Model file for the job. Use its own axes, mm. A direction names the side the tool comes from. Coordinates: 2 decimals unless noted, no trailing zeros. Write each loop counter-clockwise with the first axis right and the second up, starting at its lowest first coordinate (ties: lowest second). Pieces come first, ordered by that corner, then holes. Notation, with made-up numbers: M -22.75,50 L -0.75,50 A17 cw -0.75,63 Z; hole C -19.5,77.25 d5. An arc over 180 degrees is marked long. Answer in a Markdown table with one row per item. Add a question column.
```python
from build123d import *

# Parameters (mm, degrees)
SALIENTE_EXTRUIR1_DEPTH = 11.5
CORTAR_EXTRUIR1_START   = -5
CROQUIS2_R              = 2.1
CORTAR_EXTRUIR1_DEPTH   = 5
CROQUIS3_R              = 4.5
CORTAR_EXTRUIR2_DEPTH   = 0.5
CROQUIS4_R              = 3
CORTAR_EXTRUIR3_DEPTH   = 0.2
CROQUIS5_R              = 2.1
CROQUIS5_R_2            = 1.6
SALIENTE_EXTRUIR2_DEPTH = 0.6
CORTAR_EXTRUIR5_DEPTH   = 11.5


with BuildPart() as part:
    # Croquis1 → Saliente-Extruir1 (new body)
    with BuildSketch(Plane.XY):
        Polygon((-89.253382482, -13.336480186), (-89.253382482, 19.863519814), (-87.853382482, 19.863519814), (-87.853382482, 16.863519814), (-84.253382482, 16.863519814), (-84.253382482, 10.863519814), (-87.853382482, 10.863519814), (-87.853382482, -10.336480186), (-86.853382482, -10.336480186), (-86.853382482, -13.336480186), align=None)
    extrude(amount=SALIENTE_EXTRUIR1_DEPTH)

    # Croquis2 → Cortar-Extruir1 (cut)
    with BuildSketch(Plane(origin=(-84.253382482, 0, 0), x_dir=(0, 0, -1), z_dir=(1, 0, 0)).offset(CORTAR_EXTRUIR1_START)):
        with Locations((-5.75, 13.863519814)):
            Circle(CROQUIS2_R)
        with Locations((-5.75, -4.336480186)):
            Circle(CROQUIS2_R)
    extrude(amount=CORTAR_EXTRUIR1_DEPTH, mode=Mode.SUBTRACT)

    # Croquis3 → Cortar-Extruir2 (cut)
    with BuildSketch(Plane(origin=(-87.853382482, 0, 0), x_dir=(0, 0, -1), z_dir=(1, 0, 0))):
        with Locations((-5.75, -4.336480186)):
            Circle(CROQUIS3_R)
    extrude(amount=-CORTAR_EXTRUIR2_DEPTH, mode=Mode.SUBTRACT)

    # Croquis4 → Cortar-Extruir3 (cut)
    with BuildSketch(Plane.ZY.offset(89.253382482)):
        with Locations((5.75, 13.863519814)):
            Circle(CROQUIS4_R)
    extrude(amount=-CORTAR_EXTRUIR3_DEPTH, mode=Mode.SUBTRACT)

    # Croquis5 → Saliente-Extruir2 (add)
    with BuildSketch(Plane.ZY.offset(89.053382482)):
        with Locations((5.75, 13.863519814)):
            Circle(CROQUIS5_R)
        with Locations((5.75, 13.863519814)):
            Circle(CROQUIS5_R_2, mode=Mode.SUBTRACT)
    extrude(amount=-SALIENTE_EXTRUIR2_DEPTH)

    # Croquis6 → Cortar-Extruir5 (cut)
    with BuildSketch(Plane.XY.offset(11.5)):
        with BuildLine():
            ThreePointArc((-78.686236851, 13.786596737), (-81.253382482, 29.363519814), (-83.820528112, 13.786596737))
            ThreePointArc((-83.820528112, 13.786596737), (-81.253382482, 2.363519814), (-78.686236851, 13.786596737))
        make_face()
    extrude(amount=-CORTAR_EXTRUIR5_DEPTH, mode=Mode.SUBTRACT)


solid = part.part
```
1) Slice it at C-C (z = 2.25). Give the cut face in (x, y).
2) Drill centre lines: probe 1 along Y at (x, z) = (-89.2, 5.75); probe 2 along Z at (x, y) = (-87.7, 14); probe 3 along X at (y, z) = (1, 6.75). Where is each one in solid material? Low to high.
3) Flat gauge pins, fed straight in: pin 1 Ø5 at (y, z) = (13.86, 5.75) entering from -X; pin 2 Ø0.8 at (x, z) = (-87, 7.5) entering from +Y; pin 3 Ø3 at (x, z) = (-85, 9) entering from +Y. Where does each tip first touch, or does it go through?
4) Slice it at B-B (x = -85.3). Give the cut face in (y, z).
5) Slice it at D-D (y = 7.5). Give the cut face in (x, z), then the cut area to 3 significant figures.
6) Two-plate mould, pull along Y, no slides. Class faces 5 (the face through (-87.47, 16.33, 5.83)), 6 (the face through (-88.1, -1.3, 9.07)), 7 (the face through (-88.2, 4.6, 0)): released by +Y, released by -Y, zero draft, split by the parting line, or undercut.
7) Which spindle directions (+Z, -Z, +X, -X, +Y, -Y) get a long thin tool onto all of the face, cutting with end or side? Do faces 1 (the face through (-88.353, -2, 5)), 2 (the face through (-89.053, 12.6, 7)), 3 (the face through (-87, 10.864, 6)), 4 (the face through (-86.853, -12, 6)). Say none if no direction does.
8) Slice it at A-A (z = 5.75). Give the cut face in (x, y), then the cut area to 3 significant figures.
Ans:
| question | item | result |
|---|---|---|
| 1 | outline | M -89.25,-13.34 L -86.85,-13.34 L -86.85,-10.34 L -87.85,-10.34 L -87.85,-7.16 L -88.35,-7.16 L -88.35,-1.51 L -87.85,-1.51 L -87.85,10.86 L -86.71,10.86 A6 cw -84.25,13.56 L -84.25,13.95 A8 cw -89.11,19.86 L -89.25,19.86 Z |
| 2 | probe 1 | y = -13.34 to -6.44, -2.24 to 10.86, 16.86 to 19.86 |
| 2 | probe 2 | z = 0 to 3.65, 7.85 to 11.5 |
| 2 | probe 3 | x = -89.25 to -87.85 |
| 3 | pin 1 | stops at x = -89.05 |
| 3 | pin 2 | stops at y = 16.24 |
| 3 | pin 3 | stops at y = 15.32 |
| 4 | outline | M 12.79,0 L 14.46,0 L 14.46,3.74 A2.1 cw 12.79,3.94 Z; M 12.79,7.56 A2.1 cw 14.46,7.76 L 14.46,11.5 L 12.79,11.5 Z |
| 5 | outline | M -89.25,0 L -87.85,0 L -87.85,11.5 L -89.25,11.5 Z |
| 5 | area | 16.1 mm2 |
| 6 | face 5 | released by +Y |
| 6 | face 6 | undercut |
| 6 | face 7 | zero draft |
| 7 | face 1 | +X |
| 7 | face 2 | -X |
| 7 | face 3 | +Z, -Z, +X |
| 7 | face 4 | +Z, -Z, +X, -Y |
| 8 | outline | M -89.25,-13.34 L -86.85,-13.34 L -86.85,-10.34 L -87.85,-10.34 L -87.85,-8.84 L -88.35,-8.84 L -88.35,-6.44 L -89.25,-6.44 Z; M -89.25,-2.24 L -88.35,-2.24 L -88.35,0.16 L -87.85,0.16 L -87.85,10.86 L -86.71,10.86 A6 cw -86.2,11.76 L -88.45,11.76 L -88.45,12.26 L -89.05,12.26 L -89.05,10.86 L -89.25,10.86 Z; M -89.25,16.86 L -89.05,16.86 L -89.05,15.46 L -88.45,15.46 L -88.45,15.96 L -87.16,15.96 A8 cw -89.11,19.86 L -89.25,19.86 Z |
| 8 | area | 34.8 mm2 |
